from build123d import *

# Parameters (mm, degrees)
SKETCH1_W                = 12
SKETCH1_H                = 10
SKETCH1_R                = 2.025
BOSS_EXTRUDE1_DEPTH      = 2
SKETCH2_R                = 0.8
SKETCH2_W                = 8.05
SKETCH2_H                = 1.05
CUT_EXTRUDE1_DEPTH       = 2
SKETCH3_W                = 6.1
SKETCH3_H                = 1.9
BOSS_EXTRUDE2_DEPTH      = 1
M1_6_TAPPED_HOLE1_REACH  = 13.185
M1_6_TAPPED_HOLE1_BORE_R = 0.625
M1_6_TAPPED_HOLE2_D      = 1.25


with BuildPart() as part:
    # Sketch1 → Boss-Extrude1 (new body)
    with BuildSketch(Plane(origin=(0, 0, 0), x_dir=(1, 0, 0), z_dir=(0, 1, 0))):
        Rectangle(SKETCH1_W, SKETCH1_H)
        with Locations(Location((0, 0, 0), (0, 0, 270))):
            Circle(SKETCH1_R, mode=Mode.SUBTRACT)
    extrude(amount=BOSS_EXTRUDE1_DEPTH)

    # Sketch2 → Cut-Extrude1 (cut)
    with BuildSketch(Plane(origin=(0, 2, 0), x_dir=(1, 0, 0), z_dir=(0, 1, 0))):
        with Locations(Location((3.89097221, 2.724488073, 0), (0, 0, 270))):
            Circle(SKETCH2_R)
        with Locations(Location((-3.89097221, -2.724488073, 0), (0, 0, 270))):
            Circle(SKETCH2_R)
        with Locations((0, 4.475)):
            Rectangle(SKETCH2_W, SKETCH2_H)
        with Locations((0, -4.475)):
            Rectangle(SKETCH2_W, SKETCH2_H)
    extrude(amount=-CUT_EXTRUDE1_DEPTH, mode=Mode.SUBTRACT)

    # Sketch3 → Boss-Extrude2 (add)
    with BuildSketch(Plane(origin=(0, 2, 0), x_dir=(1, 0, 0), z_dir=(0, 1, 0))):
        with Locations((-0.975, 3)):
            Rectangle(SKETCH3_W, SKETCH3_H)
        with Locations((0.975, -3)):
            Rectangle(SKETCH3_W, SKETCH3_H)
    extrude(amount=BOSS_EXTRUDE2_DEPTH)

    # M1.6 Tapped Hole1 bore → M1.6 Tapped Hole1 (cut, up to next)
    with BuildSketch(Plane.XY.offset(3.95), mode=Mode.PRIVATE) as m1_6_tapped_hole1_sk1:
        with Locations((0, 1.5)):
            Circle(M1_6_TAPPED_HOLE1_BORE_R)
    m1_6_tapped_hole1_tool1 = extrude(m1_6_tapped_hole1_sk1.sketch, amount=-M1_6_TAPPED_HOLE1_REACH, mode=Mode.PRIVATE) & part.part
    add(m1_6_tapped_hole1_tool1.solids().sort_by_distance((0, 1.5, 3.95))[0], mode=Mode.SUBTRACT)

    # M1.6 Tapped Hole2 (through all)
    with Locations(Plane(origin=(0, 0, -3.95), x_dir=(-1, 0, 0), z_dir=(0, 0, -1))):
        with Locations((0, 1.5)):
            Hole(M1_6_TAPPED_HOLE2_D / 2)


solid = part.part
Geometry check sheet. Reference: the model listing, model coordinates, mm. A direction names the side the tool comes from. Round coordinates to 2 decimals unless told otherwise and drop trailing zeros. Write each loop counter-clockwise with the first axis right and the second up, starting at its lowest first coordinate (ties: lowest second). Pieces come first, ordered by that corner, then holes. Notation, with made-up numbers: (80, 2.5) - (100, 2.5) arc R28 ccw to (100, 35.5) - close; hole circle Ø9 at (1, 4). An arc over 180 degrees is marked (long way). One line per item, written item: value.
1. Scan lines: L1, parallel to Z at x = 0.25, y = 2.8; L2, parallel to X at y = 1.65, z = -4.5 (3 decimals); L3, parallel to Y at x = 0, z = 2.65 (3 decimals). Record each from-to range of solid material in increasing order.
The answers:
L1: z = -3.95 to -2.05, 2.05 to 3.95
L2: x = -6 to -4.025, 4.025 to 6
L3: y = 0 to 0.875, 2.125 to 3
2. Set-up check for faces 4 (the face through (4.025, 2.5, 3)), 5 (the face through (0.9, 2.5, 2.05)), 6 (the face through (-2.075, 2.5, 3)): record each of +Z, -Z, +X, -X, +Y, -Y from which the full face is reachable in a straight line by a thin tool's end or side.
The answers:
face 4: +Z, -Z, +X, +Y
face 5: +X, -X, +Y
face 6: +Z, -X, +Y
3. Depth check by flat-ended pin: pin 1 Ø1 at (x, y) = (1, 0.5) entering from -Z; pin 2 Ø0.5 at (y, z) = (2.5, -3) entering from +X (3 decimals); pin 3 Ø1.7 at (x, z) = (-3, 0.5) entering from +Y. Enter the tip coordinate at first touch or a pass-through.
The answers:
pin 1: stops at z = -3.95
pin 2: stops at x = 2.075
pin 3: stops at y = 2
4. Mould release check, pull along Z, two halves, no side actions. Record for faces 1 (the face through (-1, 2.5, -2.05)), 2 (the face through (4.025, 1, 4.5)), 3 (the face through (-1, 1, -3.95)): released by +Z, released by -Z, zero draft, split by the parting line, or undercut.
The answers:
face 1: undercut
face 2: zero draft
face 3: released by -Z
5. Cross-section at D-D on x = -3.25. Record the boundary of the cut face in (y, z), and give its area (3 significant figures).
The answers:
outline: (0, -3.95) - (3, -3.95) - (3, -2.05) - (2, -2.05) - (2, 2.25) - (0, 2.25) - close; (0, 3.2) - (2, 3.2) - (2, 3.95) - (0, 3.95) - close
area: 15.8 mm^2
6. Cross-section at C-C on z = 0. Record the boundary of the cut face in (x, y) (3 decimals), and give its area (3 significant figures).
The answers:
outline: (-6, 0) - (-2.025, 0) - (-2.025, 2) - (-6, 2) - close; (2.025, 0) - (6, 0) - (6, 2) - (2.025, 2) - close
area: 15.9 mm^2
7. Cross-section at A-A on x = 0. Record the boundary of the cut face in (y, z) (3 decimals), and give its area (3 significant figures).
The answers:
outline: (0, -3.95) - (0.875, -3.95) - (0.875, -2.025) - (0, -2.025) - close; (0, 2.025) - (0.875, 2.025) - (0.875, 3.95) - (0, 3.95) - close; (2.125, -3.95) - (3, -3.95) - (3, -2.05) - (2.125, -2.05) - close; (2.125, 2.05) - (3, 2.05) - (3, 3.95) - (2.125, 3.95) - close
area: 6.69 mm^2
8. Cross-section at B-B on y = 2.6. Record the boundary of the cut face in (x, z) (3 decimals).
The answers:
outline: (-4.025, -3.95) - (2.075, -3.95) - (2.075, -2.05) - (-4.025, -2.05) - close; (-2.075, 2.05) - (4.025, 2.05) - (4.025, 3.95) - (-2.075, 3.95) - close
